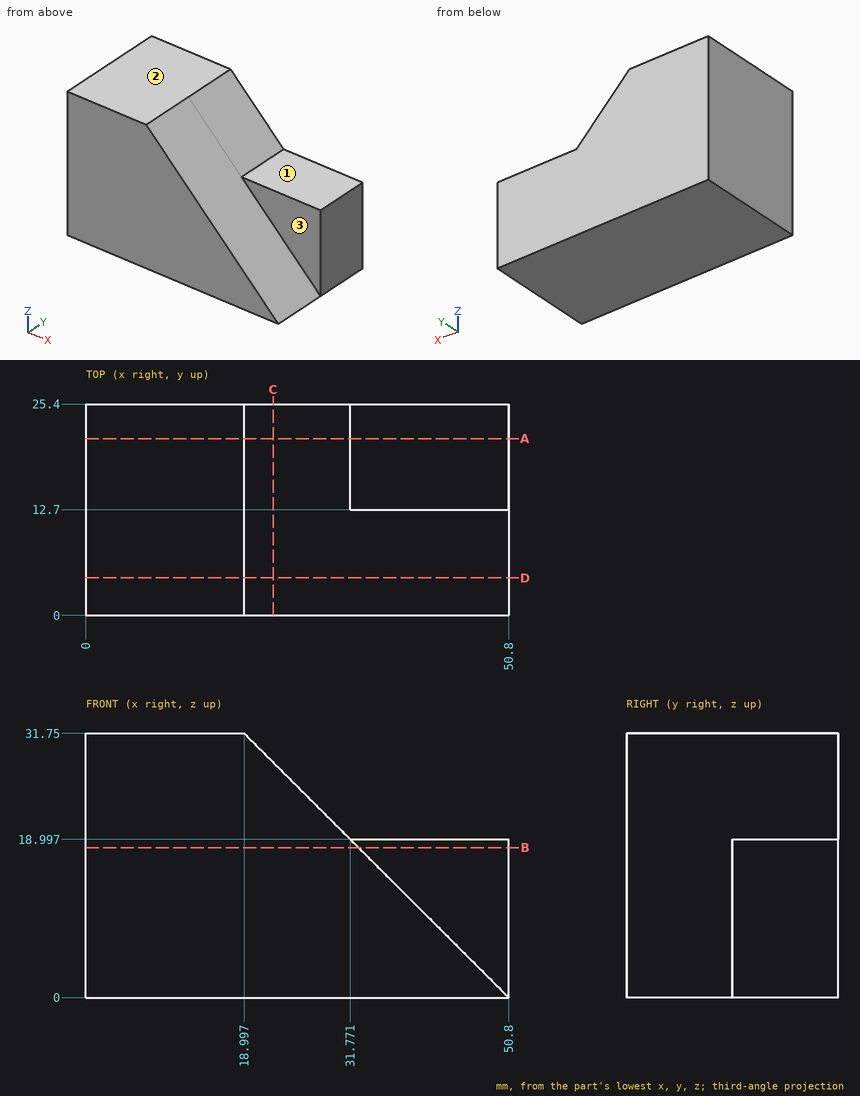
Geometry: see drawing. Coordinates: mm, zero at the bounding-box minimum. A direction names the side the tool comes from. Give positions to 0.01 mm unless a question says otherwise; leave off trailing zeros. Loops run counter-clockwise (first coordinate to the right, second up) from the corner with the lowest first, then second, coordinate; pieces in that order, holes last. Notation, with made-up numbers: (-15, -31) -> (25, -31) arc R7 ccw to (25, -22) -> close; hole circle Ø3 at (34.5, -4). An arc over 180 degrees is marked (long way). Put each result on its own line as item: value.
1. Pin query (flat end, axial travel): P1, Ø5.5, axis at x = 38, z = 7.5, coming from the -Y side; P2, Ø6.5, axis at x = 44, y = 21, coming from the +Z side; P3, Ø6, axis at x = 24, y = 7, coming from the +Z side. Return the tip coordinate at first contact, or that it passes through.
Taken from the geometry:
P1: stops at y = 0
P2: stops at z = 19
P3: stops at z = 29.75
2. Ray query, line 1 along Y through (x, z) = (40, 16.5); line 2 along Z through (x, y) = (33, 20); line 3 along Z through (x, y) = (23.5, 13.5) (1 decimal). Return the intervals inside material, ascending. Write a range as [from, to].
Taken from the geometry:
line 1: y = [12.7, 25.4]
line 2: z = [0, 19]
line 3: z = [0, 27.3]
3. Cut plane B-B (z = 18). Return the cut outline in (x, y).
Taken from the geometry:
outline: (0, 0) -> (32.77, 0) -> (32.77, 12.7) -> (50.8, 12.7) -> (50.8, 25.4) -> (0, 25.4) -> close
4. Cut plane D-D (y = 4.5). Return the cut outline in (x, z).
Taken from the geometry:
outline: (0, 0) -> (50.8, 0) -> (19, 31.75) -> (0, 31.75) -> close
5. Cut plane A-A (y = 21.25). Return the cut outline in (x, z), plus the area to 3 significant figures.
Taken from the geometry:
outline: (0, 0) -> (50.8, 0) -> (50.8, 19) -> (31.77, 19) -> (19, 31.75) -> (0, 31.75) -> close
area: 1,290 mm2
6. Cut plane C-C (x = 22.5). Return the cut outline in (y, z), plus the area to 3 significant figures.
Taken from the geometry:
outline: (0, 0) -> (25.4, 0) -> (25.4, 28.25) -> (0, 28.25) -> close
area: 718 mm2
7. Set-up query: the marked faces 1, 2 and 3. Return all of +Z, -Z, +X, -X, +Y, -Y with unobstructed straight access to the full face (end or side cutting, diameter ignored); none if empty.
Taken from the geometry:
face 1: +Z, +X, +Y, -Y
face 2: +Z, +X, -X, +Y, -Y
face 3: +Z, +X, -Y
